Here's how the part is built. I have some questions about the finished solid (model axes, mm). A direction names the side the tool comes from. Round coordinates to 2 decimals unless told otherwise and drop trailing zeros. Write each loop counter-clockwise with the first axis right and the second up, starting at its lowest first coordinate (ties: lowest second). Pieces come first, ordered by that corner, then holes. Notation, with made-up numbers: (70.5, 58.5) -> (105.5, 58.5) arc R11 ccw to (105.5, 64.5) -> close; hole circle Ø5 at (87.25, 69). An arc over 180 degrees is marked (long way). Answer in a Markdown table with one row per item.
from build123d import *

# Parameters (mm, degrees)
F1_DEPTH = 3
F3_START = -14.5
F2_W     = 12.2653646395
F2_H     = 4
F3_DEPTH = 4
F5_START = 17.05
F5_DEPTH = 4


with BuildPart() as f1:
    # F0 (on Front) → F1 (new body)
    with BuildSketch(Plane.XZ):
        Polygon((18.5, 21.05), (-18.5, 21.05), (-18.5, -21.05), (-2.25, -21.05), (-2.25, -16.55), (2.25, -16.55), (2.25, -21.05), (18.5, -21.05), align=None)
    extrude(amount=F1_DEPTH)

    # F2 (on Right) → F3 (join)
    with BuildSketch(Plane.YZ.offset(F3_START)):
        with Locations((6.1326823197, 19.05)):
            Rectangle(F2_W, F2_H)
    extrude(amount=-F3_DEPTH)

    # F4 (on Top) → F5 (join)
    with BuildSketch(Plane.XY.offset(F5_START)):
        Polygon((-22.5, -3), (-18.5, -3), (-18.5, 16.2653646395), (-14.5, 16.2653646395), (-14.5, 20.2653646395), (-22.5, 20.2653646395), align=None)
    extrude(amount=F5_DEPTH)

    # F6: F1 across plane


with BuildPart() as f1_1:
    add(f1.part)
    add(f1.part.mirror(Plane.YZ))


solid = f1_1.part
1) For pin 1 (1 mm diameter, centred on x = 13.5, y = 12.5, fed in from -Z); pin 2 (6.5 mm diameter, centred on x = -18.5, y = 12.5, fed in from -Z); pin 3 (0.9 mm diameter, centred on y = -1, z = 5, fed in from -X); pin 4 (0.9 mm diameter, centred on y = -2, z = -19.5, fed in from +X), each with a flat end and sliding along its axis, tell me the tip position at first contact or that it passes through.
Response:
| item | result |
|---|---|
| pin 1 | passes through |
| pin 2 | stops at z = 17.05 |
| pin 3 | stops at x = -18.5 |
| pin 4 | stops at x = 18.5 |
2) I want a section at C-C, the plane y = 8. List the corners of the cut face in (x, z) for me.
Response:
| item | result |
|---|---|
| outline | (-22.5, 17.05) -> (-14.5, 17.05) -> (-14.5, 21.05) -> (-22.5, 21.05) -> close; (14.5, 17.05) -> (22.5, 17.05) -> (22.5, 21.05) -> (14.5, 21.05) -> close |
3) I want a section at B-B, the plane z = -18. List the corners of the cut face in (x, y) for me, and give its area (3 significant figures).
Response:
| item | result |
|---|---|
| outline | (-18.5, -3) -> (-2.25, -3) -> (-2.25, 0) -> (-18.5, 0) -> close; (2.25, -3) -> (18.5, -3) -> (18.5, 0) -> (2.25, 0) -> close |
| area | 97.5 mm^2 |
4) Which directions (+Z, -Z, +X, -X, +Y, -Y) give clear straight access to the entire face, cutting with the end or side of a thin tool? Please do faces 5 (the face through (18.5, -1, -2)), 6 (the face through (0, -1, -16.55)), 7 (the face through (-18.5, 14, 19)), 8 (the face through (-14.5, 6, 19)).
Response:
| item | result |
|---|---|
| face 5 | -Z, +X, +Y, -Y |
| face 6 | -Z, +Y, -Y |
| face 7 | +Z, -Z |
| face 8 | +Z, -Z, +Y |
5) I want a section at A-A, the plane x = -17.5. List the corners of the cut face in (y, z) for me, and give its area (3 significant figures).
Response:
| item | result |
|---|---|
| outline | (-3, -21.05) -> (0, -21.05) -> (0, 17.05) -> (12.27, 17.05) -> (12.27, 21.05) -> (-3, 21.05) -> close; (16.27, 17.05) -> (20.27, 17.05) -> (20.27, 21.05) -> (16.27, 21.05) -> close |
| area | 191 mm^2 |
6) I want a section at D-D, the plane x = -5.5. List the corners of the cut face in (y, z) for me.
Response:
| item | result |
|---|---|
| outline | (-3, -21.05) -> (0, -21.05) -> (0, 21.05) -> (-3, 21.05) -> close |
7) I need wall thicknesses on line 1 (X direction, y = -1.5, z = -19); line 2 (Z direction, x = -20, y = -2); line 3 (Y direction, x = 2, z = 15). Which ranges of each line are inside material? Lowest first, please. Write a range as [from, to].
Response:
| item | result |
|---|---|
| line 1 | x = [-18.5, -2.25], [2.25, 18.5] |
| line 2 | z = [17.05, 21.05] |
| line 3 | y = [-3, 0] |
8) We'd pull the mould along Y, two halves only. Please class faces 1 (the face through (18, 20.265, 19)), 2 (the face through (-22.5, 9, 19)), 3 (the face through (17, 16.265, 19)), 4 (the face through (0, -3, 0)): +Y half, -Y half, draft (parallel to the pull), parting line (faces both ways), or undercut.
Response:
| item | result |
|---|---|
| face 1 | +Y half |
| face 2 | draft |
| face 3 | undercut |
| face 4 | -Y half |
